from build123d import *

# Parameters (mm, degrees)
F0_R     = 45
F1_DEPTH = 12.7
F2_R     = 45
F2_R_2   = 41
F3_DEPTH = 38.1
F4_R     = 2.38125
F5_DEPTH = 79.502
F6_R     = 2.38125
F7_DEPTH = 25.4
F8_R     = 12.7
F9_DEPTH = 25.4


with BuildPart() as f1:
    # F0 (on Top) → F1 (new body)
    with BuildSketch(Plane.XY):
        Circle(F0_R)
    extrude(amount=F1_DEPTH)

    # F2 (on face) → F3 (join)
    with BuildSketch(Plane.XY.offset(12.7)):
        Circle(F2_R)
        Circle(F2_R_2, mode=Mode.SUBTRACT)
    extrude(amount=F3_DEPTH)

    # F4 (on Front) → F5 (cut)
    with BuildSketch(Plane.XZ):
        with Locations((0, 25.4)):
            Circle(F4_R)
    extrude(amount=F5_DEPTH, mode=Mode.SUBTRACT)

    # F6 (on face) → F7 (cut)
    with BuildSketch(Plane.XY.offset(12.7)):
        with Locations((-25.4, 0)):
            Circle(F6_R)
        with Locations((25.4, 0)):
            Circle(F6_R)
    extrude(amount=-F7_DEPTH, mode=Mode.SUBTRACT)

    # F8 (on face) → F9 (cut)
    with BuildSketch(Plane.XY.offset(12.7)):
        with Locations((0, 10.16)):
            Circle(F8_R)
    extrude(amount=-F9_DEPTH, mode=Mode.SUBTRACT)


solid = f1.part
Verification items for the finished model (mm, model axes). A direction names the side the tool comes from. Coordinates: 2 decimals unless noted, no trailing zeros. Loops run counter-clockwise (first coordinate to the right, second up) from the corner with the lowest first, then second, coordinate; pieces in that order, holes last. Notation, with made-up numbers: (38.25, 7) -> (90.25, 7) arc R23 ccw to (90.25, 21) -> close; hole circle Ø1 at (-10, -11). An arc over 180 degrees is marked (long way). Answer as a JSON object with one key per item and string values. Group by question number.
Item 1: Tool access check on faces 1 (the flat face through (-10, -40, 50.8)), 2 (the flat face through (-1, -9, 12.7)), 3 (the cylindrical face through (-1.755, -42.937, 27.009)). Record the directions out of +Z, -Z, +X, -X, +Y, -Y that give a thin tool (end or side, any length) a straight path to the whole face; none if there is none.
Item 2: Sectioned sample at D-D on x = 11. Record the boundary of the cut face in (y, z), plus the area to 3 significant figures.
Item 3: Scan lines: probe 1 along X at (y, z) = (-0.5, 43); probe 2 along Z at (x, y) = (0, -43); probe 3 along Y at (x, z) = (-24, 37.5). Record each from-to range of solid material in increasing order.
Item 4: Sectioned sample at C-C on y = 10.16. Record the boundary of the cut face in (x, z).
Item 5: Sectioned sample at A-A on x = 0. Record the boundary of the cut face in (y, z), plus the area to 3 significant figures.
Item 6: Mould release check, pull along X, two halves, no side actions. Record for faces 4 (the cylindrical face through (20.765, -39.923, 25.044)), 5 (the flat face through (-1, -9, 0)), 6 (the cylindrical face through (-2.75, -2.24, 6.44)), 7 (the cylindrical face through (-9, -40, 31)): +X half, -X half, draft (parallel to the pull), parting line (faces both ways), or undercut.
Item 7: Sectioned sample at B-B on y = 0. Record the boundary of the cut face in (x, z), plus the area to 3 significant figures.
Item 8: Depth check by flat-ended pin: pin 1 (12 mm diameter, centred on x = -11, z = 39, fed in from -Y); pin 2 (8 mm diameter, centred on y = 20, z = 17, fed in from +X); pin 3 (1 mm diameter, centred on y = -20, z = 30, fed in from -X). Enter the tip coordinate at first touch or a pass-through.
Evaluation:
{
 "1": {"face 1": "+Z, +X, -X, +Y, -Y", "face 2": "+Z", "face 3": "-Y"},
 "2": {"outline": "(-43.63, 0) -> (3.81, 0) -> (3.81, 12.7) -> (-39.5, 12.7) -> (-39.5, 50.8) -> (-43.63, 50.8) -> close; (16.51, 0) -> (43.63, 0) -> (43.63, 50.8) -> (39.5, 50.8) -> (39.5, 12.7) -> (16.51, 12.7) -> close", "area": "1,260 mm²"},
 "3": {"probe 1": "x = -45 to -41, 41 to 45", "probe 2": "z = 0 to 23.02, 27.78 to 50.8", "probe 3": "y = -38.07 to -33.24, 33.24 to 38.07"},
 "4": {"outline": "(-43.84, 0) -> (-12.7, 0) -> (-12.7, 12.7) -> (-39.72, 12.7) -> (-39.72, 50.8) -> (-43.84, 50.8) -> close; (12.7, 0) -> (43.84, 0) -> (43.84, 50.8) -> (39.72, 50.8) -> (39.72, 12.7) -> (12.7, 12.7) -> close"},
 "5": {"outline": "(-45, 0) -> (-2.54, 0) -> (-2.54, 12.7) -> (-41, 12.7) -> (-41, 23.02) -> (-45, 23.02) -> close; (-45, 27.78) -> (-41, 27.78) -> (-41, 50.8) -> (-45, 50.8) -> close; (22.86, 0) -> (45, 0) -> (45, 50.8) -> (41, 50.8) -> (41, 12.7) -> (22.86, 12.7) -> close", "area": "1,110 mm²"},
 "6": {"face 4": "parting line", "face 5": "draft", "face 6": "undercut", "face 7": "undercut"},
 "7": {"outline": "(-45, 0) -> (-27.78, 0) -> (-27.78, 12.7) -> (-41, 12.7) -> (-41, 50.8) -> (-45, 50.8) -> close; (-23.02, 0) -> (-7.62, 0) -> (-7.62, 12.7) -> (-23.02, 12.7) -> close; (7.62, 0) -> (23.02, 0) -> (23.02, 12.7) -> (7.62, 12.7) -> close; (27.78, 0) -> (45, 0) -> (45, 50.8) -> (41, 50.8) -> (41, 12.7) -> (27.78, 12.7) -> close", "area": "1,130 mm²"},
 "8": {"pin 1": "stops at y = -44.72", "pin 2": "stops at x = 42.06", "pin 3": "stops at x = -40.56"}
}
